Autodesk Inventor part; units mm, degrees
ref_plane "YZ Plane" through (0, 0, 0) normal (1, 0, 0) x (0, 1, 0)
ref_plane "XZ Plane" through (0, 0, 0) normal (0, 1, 0) x (-1, 0, 0)
ref_plane "XY Plane" through (0, 0, 0) normal (0, 0, 1) x (1, 0, 0)
sketch "スケッチ1" plane through (0, 0, 0) normal (0, 0, 1) x (1, 0, 0)
  line L0 (-10, -30) -> (10, -30)
  line L1 (10, -30) -> (10, 30)
  line L2 (10, 30) -> (-10, 30)
  line L3 (-10, 30) -> (-10, -30)
  line L4 (-10, -30) -> (10, 30) construction
  line L5 (10, -30) -> (-10, 30) construction
  point P0 (0, 0)
  dimension "d0" = 20
  dimension "d1" = 60
extrude "押し出し1" add sketch "スケッチ1" along normal blind 10
chamfer "面取り1" distance 5 angle 45 2 edges at (0, 30, 10) (0, -30, 10)
fillet "フィレット1" radius 2 4 edges at (0, 30, 5) (0, 25, 10) (0, -25, 10) (0, -30, 5)
chamfer "面取り2" distance 2 angle 45 18 edges at (10, 0, 10) (10, 24.9369, 9.8478) (10, 27.5, 7.5) (10, 29.8478, 4.9369) (10, 30, 2.0858) (10, -24.9369, 9.8478) (10, -27.5, 7.5) (10, -29.8478, 4.9369) (10, -30, 2.0858) (-10, 0, 10) (-10, -24.9369, 9.8478) (-10, -27.5, 7.5) (-10, -29.8478, 4.9369) (-10, -30, 2.0858) (-10, 24.9369, 9.8478) (-10, 27.5, 7.5) (-10, 29.8478, 4.9369) (-10, 30, 2.0858)
sketch "スケッチ2" plane through (0, 0, 10) normal (0, 0, 1) x (1, 0, 0)
  line L0 (-8, -24.1716) -> (-8, 24.1716)
  line L1 (8, -24.1716) -> (-8, -24.1716)
  line L2 (8, 24.1716) -> (8, -24.1716)
  line L3 (-8, 24.1716) -> (8, 24.1716)
  point P0 (0, 0)
  point P1 (0, 20)
  point P2 (0, -20)
  dimension "d11" = 40
  dimension "d12" = 20
hole "穴1" at (0, 20, 10) at (0, -20, 10) direction (0, 0, -1) diameter 4.2 depth 21.5 counterbore diameter 8 counterbore depth 4.2
chamfer "面取り3" distance 1 angle 45 2 edges at (0, 24, 10) (0, -16, 10)
properties part number "Flame_Cover_A"
The listing builds one solid part. Answer for the finished solid, in the listing's coordinates (mm). Coordinates: 2 decimals unless noted, no trailing zeros. Write each loop counter-clockwise with the first axis right and the second up, starting at its lowest first coordinate (ties: lowest second). Pieces come first, ordered by that corner, then holes. Notation, with made-up numbers: (-25, 61) - (-10, 61) arc R26 cw to (-10, 87) - close; hole circle Ø5 at (19, 79.5). An arc over 180 degrees is marked (long way). Answer as CSV lines item,"result".
1. Find section B-B (z = 2). Give the vertices of the cut face in (x, y).
Computed values:
outline,"(-10, -28) - (-8, -30) - (8, -30) - (10, -28) - (10, 28) - (8, 30) - (-8, 30) - (-10, 28) - close; hole circle Ø4.2 at (0, -20); hole circle Ø4.2 at (0, 20)"
2. Find section A-A (y = -20). Give the vertices of the cut face in (x, z).
Computed values:
outline,"(-10, 0) - (-2.1, 0) - (-2.1, 5.8) - (-4, 5.8) - (-4, 9) - (-5, 10) - (-8, 10) - (-10, 8) - close; (2.1, 0) - (10, 0) - (10, 8) - (8, 10) - (5, 10) - (4, 9) - (4, 5.8) - (2.1, 5.8) - close"
3. Find section C-C (x = 0). Give the vertices of the cut face in (y, z).
Computed values:
outline,"(-30, 0) - (-22.1, 0) - (-22.1, 5.8) - (-24, 5.8) - (-24, 9) - (-24.87, 9.87) arc R2 ccw to (-25.59, 9.41) - (-29.41, 5.59) arc R2 ccw to (-30, 4.17) - close; (-17.9, 0) - (17.9, 0) - (17.9, 5.8) - (16, 5.8) - (16, 9) - (15, 10) - (-15, 10) - (-16, 9) - (-16, 5.8) - (-17.9, 5.8) - close; (22.1, 0) - (30, 0) - (30, 4.17) arc R2 ccw to (29.41, 5.59) - (25.59, 9.41) arc R2 ccw to (24.87, 9.87) - (24, 9) - (24, 5.8) - (22.1, 5.8) - close"
4. Find section D-D (y = -6). Give the vertices of the cut face in (x, z).
Computed values:
outline,"(-10, 0) - (10, 0) - (10, 8) - (8, 10) - (-8, 10) - (-10, 8) - close"
5. Given P1, Ø5, axis at x = 0, y = 20, coming from the +Z side; P2, Ø6, axis at x = -3.5, z = 8, coming from the -Y side; P3, Ø5, axis at x = 4.5, z = 9, coming from the +Y side, each flat-ended and moving along its own axis, determine where each tip first touches the part or whether it passes through.
Computed values:
P1,"stops at z = 5.8"
P2,"stops at y = -29.82"
P3,"stops at y = 28.5"
6. Straight lines are drawn through the part: line 1 (X direction, y = -20, z = 7.8); line 2 (Y direction, x = 0, z = 1.2); line 3 (X direction, y = 20, z = 3). For each, find the intervals that lie inside material, in ascending order. Write a range as [from, to].
Computed values:
line 1,"x = [-10, -4], [4, 10]"
line 2,"y = [-30, -22.1], [-17.9, 17.9], [22.1, 30]"
line 3,"x = [-10, -2.1], [2.1, 10]"
7. Determine the mould class of faces 1 (the flat face through (-9, -29, 2)), 2 (the flat face through (2, 18, 5.8)), 3 (the cylindrical face through (-0.112, 29.844, 4.947)), 4 (the cylindrical face through (2.4, 23.2, 7.4)) for opening direction Y: +Y half, -Y half, draft (parallel to the pull), parting line (faces both ways), or undercut.
Computed values:
face 1,"-Y half"
face 2,"undercut"
face 3,"+Y half"
face 4,"undercut"
